Geometry: see drawing. Coordinates: mm, zero at the bounding-box minimum. A direction names the side the tool comes from. Round coordinates to 2 decimals unless told otherwise and drop trailing zeros. Write each loop counter-clockwise with the first axis right and the second up, starting at its lowest first coordinate (ties: lowest second). Pieces come first, ordered by that corner, then holes. Notation, with made-up numbers: M 12.5,5.5 L 56.5,5.5 A15 ccw 56.5,15.5 Z; hole C 17,-5 d9. An arc over 180 degrees is marked long. Use one line per item in the form item = value. Start each with the question number.
Item 1: Section query C-C (y = 67.5). Return loops of the section in (x, z) (1 decimal).
Item 2: Reachability of the marked faces 1 and 2 from +Z, -Z, +X, -X, +Y, -Y: full face, straight path, thin tool, end or side. Return the list, or none.
Item 3: Section query D-D (z = 5). Return loops of the section in (x, y).
Item 4: Section query B-B (x = 60). Return loops of the section in (y, z), and give its area (3 significant figures).
Item 5: Section query A-A (z = 21.5). Return loops of the section in (x, y), and give its area (3 significant figures).
Item 6: Pull-direction query (Y, two-part tool) for the marked faces 3 and 4; classes: pulls with the +Y half, pulls with the -Y half, needs draft (parallel to the pull), parting line crosses it, or undercut.
Item 7: Ray query, probe 1 along Y at (x, z) = (60, 29); probe 2 along Z at (x, y) = (56.5, 26); probe 3 along X at (y, z) = (62, 20.5). Return the intervals inside material, ascending.
Item 8: Pin query (flat end, axial travel): pin 1 Ø12 at (y, z) = (51.5, 31.5) entering from -X; pin 2 Ø10 at (x, y) = (68.5, 61.5) entering from +Z; pin 3 Ø12 at (x, z) = (80, 5) entering from +Y. Return the tip coordinate at first contact, or that it passes through.
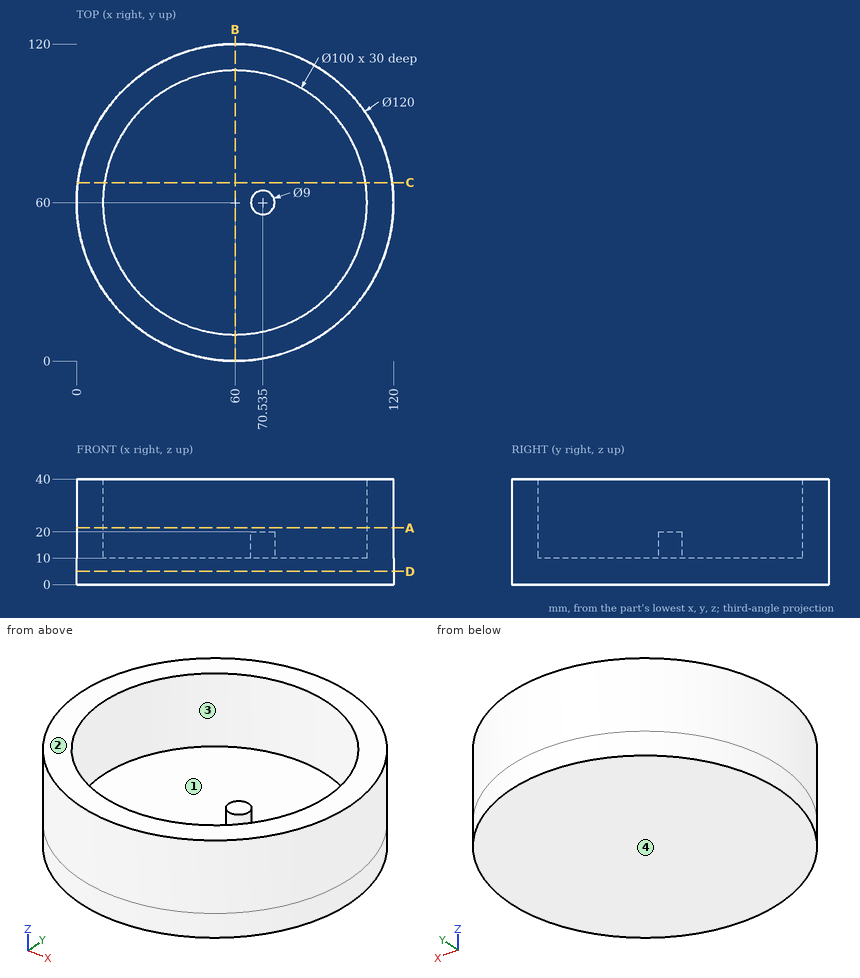
Working result:
q1.outline = M 0.5,0 L 119.5,0 L 119.5,40 L 109.4,40 L 109.4,10 L 10.6,10 L 10.6,40 L 0.5,40 Z
q2.face_1 = +Z
q2.face_2 = +Z, +X, -X, +Y, -Y
q3.outline = C 60,60 d120
q4.outline = M 0,0 L 120,0 L 120,40 L 110,40 L 110,10 L 10,10 L 10,40 L 0,40 Z
q4.area = 1,800 mm²
q5.outline = C 60,60 d120; hole C 60,60 d100
q5.area = 3,460 mm²
q6.face_3 = undercut
q6.face_4 = needs draft
q7.probe_1 = 0 to 10, 110 to 120
q7.probe_2 = 0 to 10
q7.probe_3 = 0.03 to 10.04, 109.96 to 119.97
q8.pin_1 = 0.05
q8.pin_2 = 20
q8.pin_3 = 118.34
